```python
from build123d import *

# Parameters (mm, degrees)
SKETCH_W        = 330
SKETCH_H        = 90
PAD_DEPTH       = 260
SKETCH001_W     = 320
SKETCH001_H     = 80
POCKET_DEPTH    = 250
SKETCH002_W     = 16
SKETCH002_H     = 260
PAD001_DEPTH    = 100
SKETCH003_R     = 2.625
POCKET001_DEPTH = 105
FILLET_R        = 5
FILLET001_R     = 5
FILLET002_R     = 5
FILLET003_R     = 2
FILLET004_R     = 1
FILLET005_R     = 1
FILLET006_R     = 1
FILLET007_R     = 1
SKETCH004_W     = 298
SKETCH004_H     = 5
PAD002_DEPTH    = 100
FILLET008_R     = 1
SKETCH005_W     = 390
SKETCH005_H     = 230
POCKET002_DEPTH = 145
SKETCH006_W     = 165
SKETCH006_H     = 230
POCKET003_DEPTH = 300


with BuildPart() as part:
    # Sketch → Pad (new body)
    with BuildSketch(Plane.XY):
        with Locations((165, 45)):
            Rectangle(SKETCH_W, SKETCH_H)
    extrude(amount=PAD_DEPTH)

    # Sketch001 (on Face6 of Pad) → Pocket (cut)
    with BuildSketch(Plane.XY.offset(260)):
        with Locations((165, 45)):
            Rectangle(SKETCH001_W, SKETCH001_H)
    extrude(amount=-POCKET_DEPTH, mode=Mode.SUBTRACT)

    # Sketch002 (on Face1 of Pocket) → Pad001 (join)
    with BuildSketch(Plane.XZ):
        with Locations((8, 130)):
            Rectangle(SKETCH002_W, SKETCH002_H)
        with Locations((322, 130)):
            Rectangle(SKETCH002_W, SKETCH002_H)
    extrude(amount=PAD001_DEPTH)

    # Sketch003 (on Face18 of Pad001) → Pocket001 (cut)
    with BuildSketch(Plane.XZ.offset(100)):
        with Locations((15, 40)):
            Circle(SKETCH003_R)
        with Locations((315, 40)):
            Circle(SKETCH003_R)
        with Locations((15, 120)):
            Circle(SKETCH003_R)
        with Locations((315, 120)):
            Circle(SKETCH003_R)
        with Locations((15, 200)):
            Circle(SKETCH003_R)
        with Locations((315, 200)):
            Circle(SKETCH003_R)
        with Locations((15, 255)):
            Circle(SKETCH003_R)
        with Locations((315, 255)):
            Circle(SKETCH003_R)
    extrude(amount=-POCKET001_DEPTH, mode=Mode.SUBTRACT)

    # Fillet
    fillet_edges = [part.edges().sort_by_distance(p)[0] for p in [
        (0, 45, 0),
    ]]
    fillet(fillet_edges, radius=FILLET_R)

    # Fillet001
    fillet001_edges = [part.edges().sort_by_distance(p)[0] for p in [
        (330, 45, 0),
    ]]
    fillet(fillet001_edges, radius=FILLET001_R)

    # Fillet002
    fillet002_edges = [part.edges().sort_by_distance(p)[0] for p in [
        (165, 90, 0),
    ]]
    fillet(fillet002_edges, radius=FILLET002_R)

    # Fillet003
    fillet003_edges = [part.edges().sort_by_distance(p)[0] for p in [
        (0, -50, 260),
    ]]
    fillet(fillet003_edges, radius=FILLET003_R)

    # Fillet004
    fillet004_edges = [part.edges().sort_by_distance(p)[0] for p in [
        (9, -100, 260),
    ]]
    fillet(fillet004_edges, radius=FILLET004_R)

    # Fillet005
    fillet005_edges = [part.edges().sort_by_distance(p)[0] for p in [
        (16, -49.5, 260),
    ]]
    fillet(fillet005_edges, radius=FILLET005_R)

    # Fillet006
    fillet006_edges = [part.edges().sort_by_distance(p)[0] for p in [
        (321, -100, 260),
    ]]
    fillet(fillet006_edges, radius=FILLET006_R)

    # Fillet007
    fillet007_edges = [part.edges().sort_by_distance(p)[0] for p in [
        (314, -49.5, 260),
    ]]
    fillet(fillet007_edges, radius=FILLET007_R)

    # Sketch004 (on Face4 of Fillet007) → Pad002 (join)
    with BuildSketch(Plane.XZ):
        with Locations((165, 2.5)):
            Rectangle(SKETCH004_W, SKETCH004_H)
    extrude(amount=PAD002_DEPTH)

    # Fillet008
    fillet008_edges = [part.edges().sort_by_distance(p)[0] for p in [
        (165, -100, 0),
    ]]
    fillet(fillet008_edges, radius=FILLET008_R)

    # Sketch005 (on Face7 of Fillet008) → Pocket002 (cut)
    with BuildSketch(Plane(origin=(0, 0, 0), x_dir=(1, 0, 0), z_dir=(0, 0, -1))):
        with Locations((175, 0)):
            Rectangle(SKETCH005_W, SKETCH005_H)
    extrude(amount=-POCKET002_DEPTH, mode=Mode.SUBTRACT)

    # Sketch006 (on Face46 of Pocket002) → Pocket003 (cut)
    with BuildSketch(Plane.XY.offset(260)):
        with Locations((247.5, 0)):
            Rectangle(SKETCH006_W, SKETCH006_H)
    extrude(amount=-POCKET003_DEPTH, mode=Mode.SUBTRACT)


solid = part.part
```
Build history of the part. All positions in model axes, mm. A direction names the side the tool comes from. Give positions to 0.01 mm unless a question says otherwise; leave off trailing zeros. Loops run counter-clockwise (first coordinate to the right, second up) from the corner with the lowest first, then second, coordinate; pieces in that order, holes last. Notation, with made-up numbers: (-38.75, 56) -> (12.25, 56) arc R22 ccw to (12.25, 65) -> close; hole circle Ø8 at (10.25, 47). An arc over 180 degrees is marked (long way). One line per question, with ' | ' between items.
Q1. Cut at D-D, the plane y = 28. Write the cut outline in (x, z), plus the area to 3 significant figures.
Filled sheet:
outline: (0, 145) -> (5, 145) -> (5, 260) -> (2, 260) arc R2 ccw to (0, 258) -> close | area: 574 mm²
Q2. Pull direction Y, two halves, no side cores. Call faces 5 (the flat face through (165, 2, 203)), 6 (the flat face through (84, 85, 203)), 7 (the flat face through (89, 0, 202)): pulls with the +Y half, pulls with the -Y half, needs draft (parallel to the pull), parting line crosses it, or undercut.
Filled sheet:
face 5: needs draft | face 6: undercut | face 7: pulls with the -Y half
Q3. Tool access for faces 1 (the flat face through (16, -49, 171)), 2 (the flat face through (165, 87, 203)), 3 (the flat face through (5, 44, 203)), 4 (the cylindrical face through (12.378, -48.235, 200.115)): list every direction of +Z, -Z, +X, -X, +Y, -Y with a clear straight run to the whole face (end or side of a thin tool).
Filled sheet:
face 1: +Z, -Z, +X, -Y | face 2: +Z, -Z, +X, +Y, -Y | face 3: +Z, -Z, +X | face 4: -Y
Q4. Cut at A-A, the plane z = 200. Write the cut outline in (x, y) (3 decimals).
Filled sheet:
outline: (0, -99) arc R1 ccw to (1, -100) -> (12.375, -100) -> (12.375, 5) -> (5, 5) -> (5, 85) -> (165, 85) -> (165, 90) -> (5, 90) arc R5 ccw to (0, 85) -> close; (17.625, 0) -> (165, 0) -> (165, 5) -> (17.625, 5) -> close
Q5. Drop flat-ended pins along their axis: pin 1 (0.5 mm diameter, centred on y = -54.5, z = 258.5, fed in from +X); pin 2 (4 mm diameter, centred on x = 15, z = 255, fed in from -Y); pin 3 (5 mm diameter, centred on y = 12, z = 197, fed in from +X). Give the stop position or say it passes through.
Filled sheet:
pin 1: stops at x = 16 | pin 2: stops at y = 85 | pin 3: stops at x = 5
Q6. Drill centre lines: line 1 along Z through (x, y) = (15, -66.5) (3 decimals); line 2 along Y through (x, z) = (104, 224); line 3 along Y through (x, z) = (10, 161). Where is each one in solid material? Low to high. Write a range as [from, to].
Filled sheet:
line 1: z = [145, 197.375], [202.625, 252.375], [257.625, 260] | line 2: y = [0, 5], [85, 90] | line 3: y = [-100, 5], [85, 90]
Q7. Cut at C-C, the plane y = -44.5. Write the cut outline in (x, z) (3 decimals), plus the area to 3 significant figures.
Filled sheet:
outline: (0, 145) -> (16, 145) -> (16, 197.573) arc R2.625 cw (long way) to (16, 202.427) -> (16, 252.573) arc R2.625 cw (long way) to (16, 257.427) -> (16, 259) arc R1 ccw to (15, 260) -> (2, 260) arc R2 ccw to (0, 258) -> close | area: 1,810 mm²
Q8. Cut at B-B, the plane x = 133. Write the cut outline in (y, z), plus the area to 3 significant figures.
Filled sheet:
outline: (0, 145) -> (5, 145) -> (5, 260) -> (0, 260) -> close; (85, 145) -> (90, 145) -> (90, 258) arc R2 ccw to (88, 260) -> (85, 260) -> close | area: 1,150 mm²
